Input: part model. Units: mm. Frame: model coordinates. A direction names the side the tool comes from. Round coordinates to 2 decimals unless told otherwise and drop trailing zeros. Order: outer loops, then holes, each group sorted by start corner. A loop starts at its lowest first (then second) coordinate and runs counter-clockwise, first axis right, second up.
Item 1: First-contact query: pin 1 (6 mm diameter, centred on x = 28.5, z = -14, fed in from -Y); pin 2 (0.9 mm diameter, centred on x = 25, y = 7.5, fed in from +Z); pin 3 (5 mm diameter, centred on x = 17, z = -16.5, fed in from +Y). Flat tips, straight axial feed; report the tip coordinate or a pass-through.
Item 2: Cut plane C-C on z = -21.5. Output: boundary loops of the cut face in (x, y), then the cut area to 3 significant figures.
Item 3: Cut plane A-A on y = 7.5. Output: boundary loops of the cut face in (x, z), then the cut area to 4 significant figures.
Item 4: Reachability of faces 4 (the flat face through (25, 6, 0)), 5 (the flat face through (25, 13, -7.5)), 6 (the flat face through (25, 2, -7.5)) from +Z, -Z, +X, -X, +Y, -Y: full face, straight path, thin tool, end or side. Return the list, or none.
Item 5: Line query: L1, parallel to Y at x = 25, z = -19.25; L2, parallel to Z at x = 29, y = 12.25; L3, parallel to Y at x = 35, z = -15.5. Output: solid intervals per line, ascending.
Item 6: Mould query, pull axis Z, two halves, no side actions, for faces 1 (the flat face through (25, 6, -30)), 2 (the flat face through (25, 5, -15)), 3 (the flat face through (25, 15, -26)). Classes: released by +Z, released by -Z, zero draft, split by the parting line, or undercut.
Item 7: Cut plane B-B on x = 25. Output: boundary loops of the cut face in (y, z), then the cut area to 3 significant figures.
Item 8: Cut plane D-D on x = 45.5. Output: boundary loops of the cut face in (y, z).
```python
from build123d import *

# Parameters (mm, degrees)
SKETCH1_W           = 50
SKETCH1_H           = 30
BOSS_EXTRUDE1_DEPTH = 15
SKETCH2_W           = 50
SKETCH2_H           = 15
CUT_EXTRUDE1_DEPTH  = 5
SKETCH3_W           = 50
SKETCH3_H           = 15
CUT_EXTRUDE2_DEPTH  = 5
SKETCH4_R           = 0.75
CUT_EXTRUDE3_DEPTH  = 30


with BuildPart() as part:
    # Sketch1 → Boss-Extrude1 (new body)
    with BuildSketch(Plane(origin=(0, 0, 0), x_dir=(1, 0, 0), z_dir=(0, 1, 0))):
        with Locations((25, 15)):
            Rectangle(SKETCH1_W, SKETCH1_H)
    extrude(amount=BOSS_EXTRUDE1_DEPTH)

    # Sketch2 → Cut-Extrude1 (cut)
    with BuildSketch(Plane(origin=(0, 15, 0), x_dir=(1, 0, 0), z_dir=(0, 1, 0))):
        with Locations((25, 15)):
            Rectangle(SKETCH2_W, SKETCH2_H)
    extrude(amount=-CUT_EXTRUDE1_DEPTH, mode=Mode.SUBTRACT)

    # Sketch3 → Cut-Extrude2 (cut)
    with BuildSketch(Plane.XZ):
        with Locations((25, -15)):
            Rectangle(SKETCH3_W, SKETCH3_H)
    extrude(amount=-CUT_EXTRUDE2_DEPTH, mode=Mode.SUBTRACT)

    # Sketch4 → Cut-Extrude3 (cut)
    with BuildSketch(Plane.XY):
        with Locations((25, 7.5)):
            Circle(SKETCH4_R)
    extrude(amount=-CUT_EXTRUDE3_DEPTH, mode=Mode.SUBTRACT)


solid = part.part
```
From the geometry:
1. pin 1: stops at y = 5
1. pin 2: passes through
1. pin 3: stops at y = 10
2. outline: (0, 5) - (50, 5) - (50, 10) - (0, 10) - close; hole circle Ø1.5 at (25, 7.5)
2. area: 248 mm2
3. outline: (0, -30) - (24.25, -30) - (24.25, 0) - (0, 0) - close; (25.75, -30) - (50, -30) - (50, 0) - (25.75, 0) - close
3. area: 1,455 mm2
4. face 4: +Z, +X, -X, +Y, -Y
4. face 5: +X, -X, +Y
4. face 6: +X, -X, -Y
5. L1: y = 5 to 6.75, 8.25 to 10
5. L2: z = -30 to -22.5, -7.5 to 0
5. L3: y = 5 to 10
6. face 1: released by -Z
6. face 2: undercut
6. face 3: zero draft
7. outline: (0, -30) - (6.75, -30) - (6.75, 0) - (0, 0) - (0, -7.5) - (5, -7.5) - (5, -22.5) - (0, -22.5) - close; (8.25, -30) - (15, -30) - (15, -22.5) - (10, -22.5) - (10, -7.5) - (15, -7.5) - (15, 0) - (8.25, 0) - close
7. area: 255 mm2
8. outline: (0, -30) - (15, -30) - (15, -22.5) - (10, -22.5) - (10, -7.5) - (15, -7.5) - (15, 0) - (0, 0) - (0, -7.5) - (5, -7.5) - (5, -22.5) - (0, -22.5) - close
